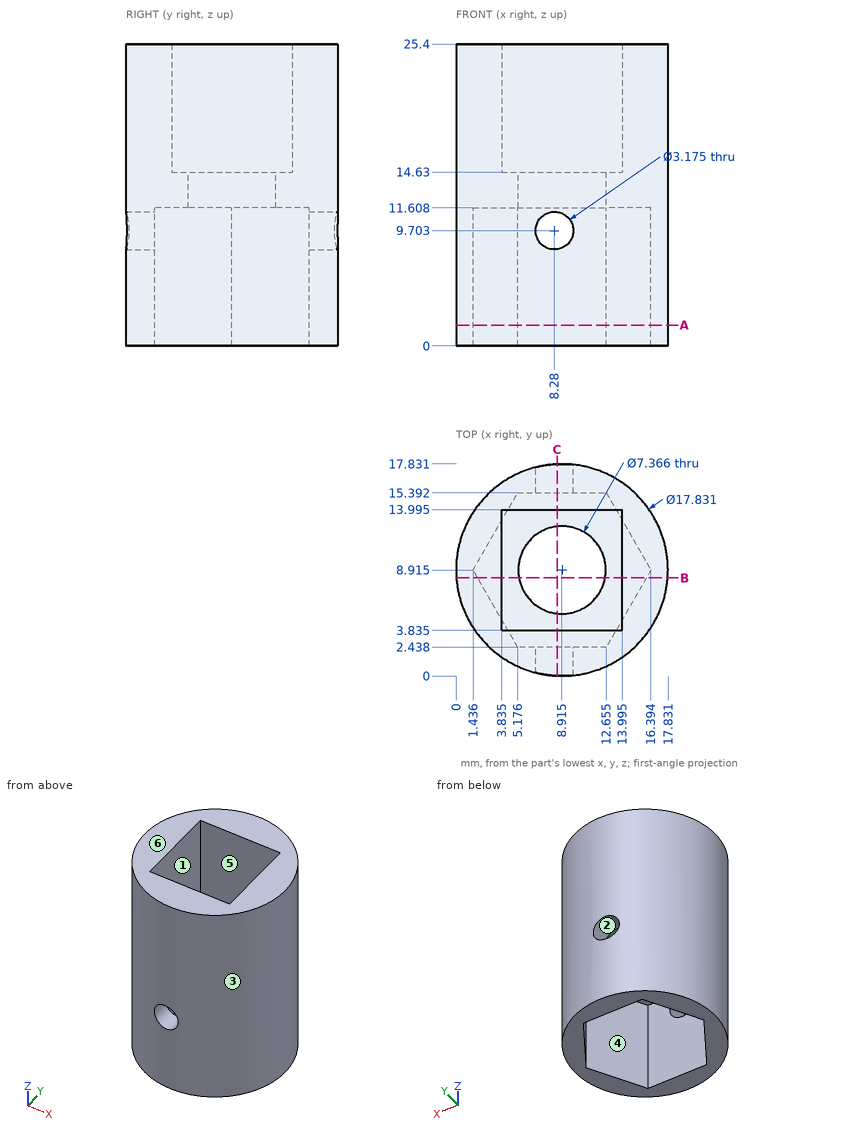
Source: three-view drawing plus pictorial views. Frame: mm from the lowest corner of the part. A direction names the side the tool comes from. Coordinates: 2 decimals unless noted, no trailing zeros. Loops run counter-clockwise (first coordinate to the right, second up) from the corner with the lowest first, then second, coordinate; pieces in that order, holes last. Notation, with made-up numbers: (-28, -13) -> (-22, -13) arc R5 cw to (-22, -7) -> close; hole circle Ø1 at (53, 69.25). An arc over 180 degrees is marked (long way). One line per item, written item: value.
(1) Cut plane B-B (y = 8.25). Output: boundary loops of the cut face in (x, z) (1 decimal), then the cut area to 3 significant figures.
Answer below:
outline: (0, 0) -> (1.8, 0) -> (1.8, 11.6) -> (5.3, 11.6) -> (5.3, 14.6) -> (3.8, 14.6) -> (3.8, 25.4) -> (0, 25.4) -> close; (12.5, 11.6) -> (16, 11.6) -> (16, 0) -> (17.8, 0) -> (17.8, 25.4) -> (14, 25.4) -> (14, 14.6) -> (12.5, 14.6) -> close
area: 156 mm2
(2) Pin query (flat end, axial travel): pin 1 Ø4 at (x, y) = (8.5, 8.5) entering from -Z; pin 2 Ø10 at (y, z) = (14.5, 18) entering from +X; pin 3 Ø6 at (y, z) = (14.5, 14) entering from +X; pin 4 Ø10 at (x, y) = (9.5, 8.5) entering from -Z. Return the tip coordinate at first contact, or that it passes through.
Answer below:
pin 1: passes through
pin 2: stops at x = 17.81
pin 3: stops at x = 17.45
pin 4: stops at z = 11.61
(3) Cut plane C-C (x = 8.5). Give the number of separate pieces and of enclosed holes in the cut face, then the cut area to 3 significant figures.
Answer below:
separate pieces: 4
enclosed holes: 0
area: 155 mm2
(4) Ray query, line 1 along Y through (x, z) = (9.25, 3.25) (1 decimal); line 2 along Y through (x, z) = (7, 12.25); line 3 along Z through (x, y) = (6.5, 3.25). Return the intervals inside material, ascending.
Answer below:
line 1: y = 0 to 2.4, 15.4 to 17.8
line 2: y = 0.21 to 5.77, 12.06 to 17.62
line 3: z = 11.61 to 25.4
(5) Set-up query: the marked faces 4, 5 and 6. Return all of +Z, -Z, +X, -X, +Y, -Y with unobstructed straight access to the full face (end or side cutting, diameter ignored); none if empty.
Answer below:
face 4: -Z
face 5: +Z
face 6: +Z, +X, -X, +Y, -Y
(6) Draft query along Y for the marked faces 1, 2 and 3. Return one class per face: pulls with the +Y half, pulls with the -Y half, needs draft (parallel to the pull), parting line crosses it, or undercut.
Answer below:
face 1: undercut
face 2: needs draft
face 3: parting line crosses it
(7) Cut plane A-A (z = 1.75). Output: boundary loops of the cut face in (x, y) (1 decimal).
Answer below:
outline: circle Ø17.8 at (8.9, 8.9); hole (1.4, 8.9) -> (5.2, 2.4) -> (12.7, 2.4) -> (16.4, 8.9) -> (12.7, 15.4) -> (5.2, 15.4) -> close
